```python
from build123d import *

# Parameters (mm, degrees)
SKETCH_2_R             = 15.938729937
CUT_EXTRUDE_1_DEPTH    = 10
HOLE_WIZARD_M6_1_D     = 5
HOLE_WIZARD_M6_1_DEPTH = 15
HOLE_WIZARD_M6_1_TIP   = 1.502151548


with BuildPart() as part:
    # 草图1 → 旋转1 (revolve)
    with BuildSketch(Plane.XY):
        with BuildLine():
            Line((0, 13.5), (0, -13.5))
            ThreePointArc((0, -13.5), (13.5, 0), (0, 13.5))
        make_face()
    revolve(axis=Axis((0, 0, 0), (0, 1, 0)))

    # 草图2 → 切除-拉伸1 (cut)
    with BuildSketch(Plane(origin=(0, 12, 0), x_dir=(-1, 0, 0), z_dir=(0, 1, 0))):
        Circle(SKETCH_2_R)
    extrude(amount=CUT_EXTRUDE_1_DEPTH, mode=Mode.SUBTRACT)

    # M6 螺纹孔1
    with Locations(Plane(origin=(0, 12, 0), x_dir=(-1, 0, 0), z_dir=(0, 1, 0))):
        with Locations((0, 0)):
            Hole(HOLE_WIZARD_M6_1_D / 2, depth=HOLE_WIZARD_M6_1_DEPTH)
            with Locations((0, 0, -(HOLE_WIZARD_M6_1_DEPTH + HOLE_WIZARD_M6_1_TIP / 2))):  # 118° drill point
                Cone(0, HOLE_WIZARD_M6_1_D / 2, HOLE_WIZARD_M6_1_TIP, mode=Mode.SUBTRACT)


solid = part.part
```
Geometry check sheet. Reference: the model listing, model coordinates, mm. Round coordinates to 2 decimals unless told otherwise and drop trailing zeros. Loops run counter-clockwise (first coordinate to the right, second up) from the corner with the lowest first, then second, coordinate; pieces in that order, holes last. Notation, with made-up numbers: M 32,88.5 L 59,88.5 A32 cw 59,120.5 Z; hole C 71.5,-4 d2. An arc over 180 degrees is marked long. Return JSON: item names as keys, results as strings. Group by question number.
(1) Section check A-A, the plane y = 7. Enter the section's corners in (x, z).
(2) Mould release check, pull along X, two halves, no side actions. Record for faces 1 (the face through (-3, 12, 0)), 2 (the face through (-0.54, 4.39, -2.44)): pulls with the +X half, pulls with the -X half, needs draft (parallel to the pull), parting line crosses it, or undercut.
(3) Section check B-B, the plane z = -5.5. Enter the section's corners in (x, y).
(4) Section check C-C, the plane x = 5. Enter the section's corners in (y, z).
(5) Go/stop test with flat-tipped pins: pin 1 (4 mm diameter, centred on x = 5.5, z = -6.5, fed in from -Y); pin 2 (5 mm diameter, centred on y = 5, z = -2, fed in from -X); pin 3 (12 mm diameter, centred on y = -6.5, z = -10.5, fed in from +X). Record where each tip stops, or that it passes through.
(6) Section check D-D, the plane y = -0.75. Enter the section's corners in (x, z).
(7) Scan lines: line 1 along Z through (x, y) = (0, 7.5); line 2 along X through (y, z) = (2.25, 0); line 3 along Z through (x, y) = (0, 8). Record each from-to range of solid material in increasing order. Write a range as [from, to].
Data:
{
 "1": {"outline": "C 0,0 d23.09; hole C 0,0 d5"},
 "2": {"face 1": "needs draft", "face 2": "undercut"},
 "3": {"outline": "M -2.83,12 A12.33 ccw long 2.83,12 Z"},
 "4": {"outline": "M 12,-3.64 L 12,3.64 A12.54 ccw long Z"},
 "5": {"pin 1": "y = -11.82", "pin 2": "x = -13.19", "pin 3": "x = 11.91"},
 "6": {"outline": "C 0,0 d26.96; hole C 0,0 d5"},
 "7": {"line 1": "[-11.22, -2.5], [2.5, 11.22]", "line 2": "[-13.31, -2.5], [2.5, 13.31]", "line 3": "[-10.87, -2.5], [2.5, 10.87]"}
}
